from build123d import *


# Read off the part's stored shape, not the designer's step: M16x2.0 Machine Threads Stud1
with BuildPart() as part:
    # Sketch1 → Revolve1 (revolve)
    with BuildSketch(Plane.XY):
        with BuildLine():
            Line((-8.5, 13.267826876), (-6.5, 13.267826876))
            Line((-6.5, 13.267826876), (-6.5, 0))
            ThreePointArc((-6.5, 0), (-6.116831152, -2.198721596), (-5.01249949, -4.138218078))
            Line((-5.01249949, -4.138218078), (-7.180291398, -6.960130418))
            ThreePointArc((-7.180291398, -6.960130418), (-9.942264304, -1.073024006), (-8.5, 5.267826876))
            Line((-8.5, 5.267826876), (-8.5, 13.267826876))
        make_face()
    revolve(axis=Axis((0, 28.261953017, 0), (0, -1, 0)))

    # M16x2.0 Machine Threads Stud1 outline → M16x2.0 Machine Threads Stud1 (revolve, cut)
    with BuildSketch(Plane.XY):
        Polygon((8.5, 13.267826876), (6.8985, 13.267826876), (8, 12.166326876), (8, 5.267826876), (8.5, 5.267826876), align=None)
    revolve(axis=Axis((0, 0, 0), (0, 1, 0)), mode=Mode.SUBTRACT)


solid = part.part
Input: part model. Units: mm. Frame: model coordinates. Give positions to 0.01 mm unless a question says otherwise; leave off trailing zeros. Order: outer loops, then holes, each group sorted by start corner. A loop starts at its lowest first (then second) coordinate and runs counter-clockwise, first axis right, second up. Notation, with made-up numbers: (-39, 51) - (11, 51) arc R8 cw to (11, 59) - close; hole circle Ø4 at (52, -10.75). An arc over 180 degrees is marked (long way). Answer as a JSON object with one key per item and string values. Group by question number.
Q1. Cut plane B-B, the plane z = 0. Output: boundary loops of the cut face in (x, y).
Q2. Line query: probe 1 along Z at (x, y) = (0, 9.5); probe 2 along X at (y, z) = (5, 1.25). Output: solid intervals per line, ascending.
Q3. Cut plane A-A, the plane x = 0. Output: boundary loops of the cut face in (y, z).
Q4. Mould query, pull axis X, two halves, no side actions, for faces 1 (the face through (-1.73, 8.67, 7.81)), 2 (the face through (5.158, 6.541, 3.955)). Classes: pulls with the +X half, pulls with the -X half, needs draft (parallel to the pull), parting line crosses it, or undercut.
Q5. First-contact query: pin 1 Ø10 at (x, y) = (-5, 2) entering from +Z; pin 2 Ø3 at (x, y) = (0.5, 10) entering from -Z; pin 3 Ø3 at (x, z) = (-4, -7.5) entering from +Y. Flat tips, straight axial feed; report the tip coordinate or a pass-through.
Q6. Cut plane C-C, the plane y = 11.5. Output: boundary loops of the cut face in (x, z), then the cut area to 3 significant figures.
Q7. Cut plane D-D, the plane y = -5. Output: boundary loops of the cut face in (x, z).
Results:
{
 "1": {"outline": "(-8.5, 5.27) arc R10 ccw to (-7.18, -6.96) - (-5.01, -4.14) arc R6.5 cw to (-6.5, 0) - (-6.5, 13.27) - (-6.9, 13.27) - (-8, 12.17) - (-8, 5.27) - close; (5.01, -4.14) - (7.18, -6.96) arc R10 ccw to (8.5, 5.27) - (8, 5.27) - (8, 12.17) - (6.9, 13.27) - (6.5, 13.27) - (6.5, 0) arc R6.5 cw to start"},
 "2": {"probe 1": "-8 to -6.5, 6.5 to 8", "probe 2": "-8.57 to -6.38, 6.38 to 8.57"},
 "3": {"outline": "(-6.96, -7.18) arc R10 ccw to (5.27, -8.5) - (5.27, -8) - (12.17, -8) - (13.27, -6.9) - (13.27, -6.5) - (0, -6.5) arc R6.5 cw to (-4.14, -5.01) - close; (-6.96, 7.18) - (-4.14, 5.01) arc R6.5 cw to (0, 6.5) - (13.27, 6.5) - (13.27, 6.9) - (12.17, 8) - (5.27, 8) - (5.27, 8.5) arc R10 ccw to start"},
 "4": {"face 1": "parting line crosses it", "face 2": "undercut"},
 "5": {"pin 1": "z = 9.99", "pin 2": "z = -8", "pin 3": "y = 13.17"},
 "6": {"outline": "circle Ø16 at (0, 0); hole circle Ø13 at (0, 0)", "area": "68.3 mm^2"},
 "7": {"outline": "circle Ø17.32 at (0, 0); hole circle Ø11.35 at (0, 0)"}
}
